For this review, take the finished solid that the model builds, in its own axes (mm). Coordinates: 2 decimals unless noted, no trailing zeros. Loops run counter-clockwise (first coordinate to the right, second up) from the corner with the lowest first, then second, coordinate; pieces in that order, holes last. Notation, with made-up numbers: (-33, 61.5) -> (23, 61.5) arc R17 ccw to (23, 72.5) -> close; hole circle Ø6 at (-1, 87). An arc over 180 degrees is marked (long way). Use a Markdown table: item, result.
from build123d import *

# Parameters (mm, degrees)
F0_W     = 100
F0_H     = 100
F0_W_2   = 80
F0_H_2   = 80
F1_DEPTH = 5
F3_D     = 5
F4_D     = 5
F4_DEPTH = 4
F4_TIP   = 1.5021515476


with BuildPart() as f1:
    # F0 (on Top) → F1 (new body)
    with BuildSketch(Plane.XY):
        with Locations((40, -40)):
            Rectangle(F0_W, F0_H)
        with Locations((40, -40)):
            Rectangle(F0_W_2, F0_H_2, mode=Mode.SUBTRACT)
        with Locations((40, -40)):
            Rectangle(F0_W_2, F0_H_2)
    extrude(amount=F1_DEPTH)

    # F3 (through all)
    with Locations(Plane(origin=(0, 0, 0), x_dir=(1, 0, 0), z_dir=(0, 0, -1))):
        with Locations((20, 9), (60, 9), (60, 71), (20, 71)):
            Hole(F3_D / 2)

    # F4
    with Locations(Plane(origin=(0, 0, 0), x_dir=(1, 0, 0), z_dir=(0, 0, -1))):
        with Locations((0, 80), (80, 80), (80, 0), (0, 0)):
            Hole(F4_D / 2, depth=F4_DEPTH)
            with Locations((0, 0, -(F4_DEPTH + F4_TIP / 2))):  # 118° drill point
                Cone(0, F4_D / 2, F4_TIP, mode=Mode.SUBTRACT)


solid = f1.part
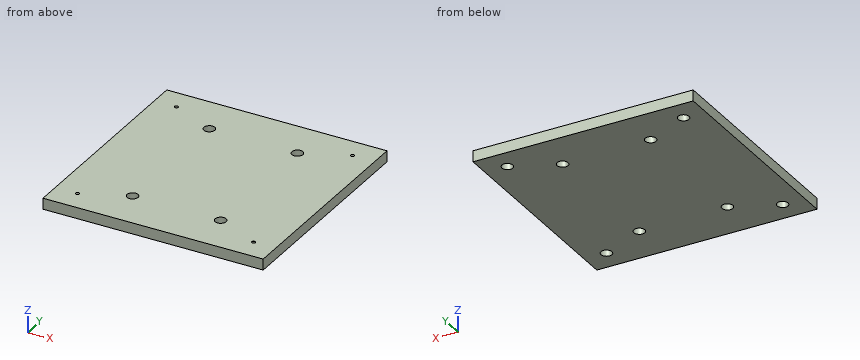
(1) Take a section at B-B on z = 0.85. State how many separate pieces and enclosed holes the cut face has, plus the area to 3 significant figures.
Found:
| item | result |
|---|---|
| separate pieces | 1 |
| enclosed holes | 8 |
| area | 9,840 mm^2 |
(2) Take a section at C-C on y = -71. Write out the cut boundary in (x, z), plus the area to 3 significant figures.
Found:
| item | result |
|---|---|
| outline | (-10, 0) -> (17.5, 0) -> (17.5, 5) -> (-10, 5) -> close; (22.5, 0) -> (57.5, 0) -> (57.5, 5) -> (22.5, 5) -> close; (62.5, 0) -> (90, 0) -> (90, 5) -> (62.5, 5) -> close |
| area | 450 mm^2 |
(3) Take a section at A-A on x = 20. Write out the cut boundary in (y, z).
Found:
| item | result |
|---|---|
| outline | (-90, 0) -> (-73.5, 0) -> (-73.5, 5) -> (-90, 5) -> close; (-68.5, 0) -> (-11.5, 0) -> (-11.5, 5) -> (-68.5, 5) -> close; (-6.5, 0) -> (10, 0) -> (10, 5) -> (-6.5, 5) -> close |
(4) For line 1 along Y through (x, z) = (20, 3.4); line 2 along X through (y, z) = (-71, 3.5); line 3 along Y through (x, z) = (80, 0.8), list the stretches that pass through material, from the lowest coordinate up.
Found:
| item | result |
|---|---|
| line 1 | y = -90 to -73.5, -68.5 to -11.5, -6.5 to 10 |
| line 2 | x = -10 to 17.5, 22.5 to 57.5, 62.5 to 90 |
| line 3 | y = -90 to -82.5, -77.5 to -2.5, 2.5 to 10 |
(5) For pin 1 Ø4 at (x, y) = (60, -9) entering from -Z; pin 2 Ø4.5 at (x, y) = (80, -80) entering from -Z, all flat-tipped, find the tip position at first contact; note any pin that passes through.
Found:
| item | result |
|---|---|
| pin 1 | passes through |
| pin 2 | stops at z = 4.15 |
